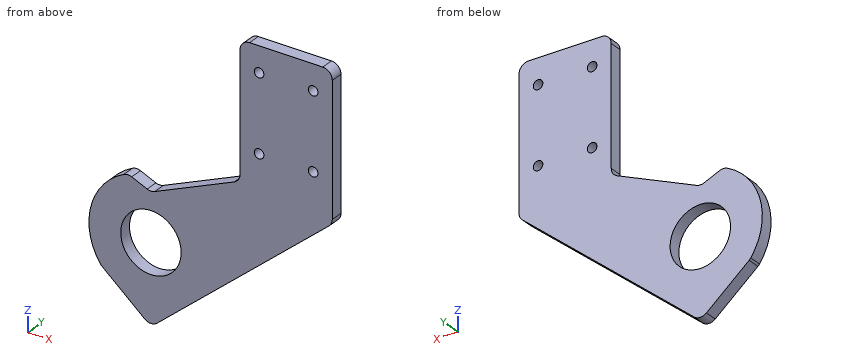
```python
from build123d import *

# Parameters (mm, degrees)
SKETCH_2_R          = 1.5
SKETCH_2_R_2        = 9.5
EXTRUDE_1_DEPTH     = 4
CUT_EXTRUDE_1_DEPTH = 124.429075185
SKETCH_6_R          = 1.5
EXTRUDE_2_DEPTH     = 4
FILLET_1_R          = 3


with BuildPart() as part:
    # 草图2 → 凸台-拉伸1 (new body)
    with BuildSketch(Plane(origin=(0, 0, 0), x_dir=(1, 0, 0), z_dir=(0, 1, 0))):
        Polygon((0, 0), (0, 60), (40, 93.908128514), (80, 60), (80, 0), (68, 0), (68, 42), (40, 54), (12, 42), (12, 0), align=None)
        with Locations(Location((6, 32, 0), (0, 0, 270))):
            Circle(SKETCH_2_R, mode=Mode.SUBTRACT)
        with Locations(Location((6, 8, 0), (0, 0, 270))):
            Circle(SKETCH_2_R, mode=Mode.SUBTRACT)
        with Locations(Location((40, 69, 0), (0, 0, 270))):
            Circle(SKETCH_2_R_2, mode=Mode.SUBTRACT)
        with Locations(Location((74, 8, 0), (0, 0, 90))):
            Circle(SKETCH_2_R, mode=Mode.SUBTRACT)
        with Locations(Location((74, 32, 0), (0, 0, 90))):
            Circle(SKETCH_2_R, mode=Mode.SUBTRACT)
    extrude(amount=EXTRUDE_1_DEPTH)

    # 草图4 → 切除-拉伸1 (cut, through all)
    with BuildSketch(Plane(origin=(0, 4, 0), x_dir=(1, 0, 0), z_dir=(0, 1, 0))):
        with BuildLine():
            Line((24.36723091, 80.656179931), (0, 60))
            Line((0, 60), (0, 0))
            Line((0, 0), (12, 0))
            Line((12, 0), (12, 42))
            Line((12, 42), (32.756034747, 50.895443463))
            ThreePointArc((32.756034747, 50.895443463), (21.23136653, 63.709593809), (24.36723091, 80.656179931))
        make_face()
    extrude(amount=-CUT_EXTRUDE_1_DEPTH, mode=Mode.SUBTRACT)

    # 草图6 → 凸台-拉伸2 (add)
    with BuildSketch(Plane(origin=(0, 4, 0), x_dir=(1, 0, 0), z_dir=(0, 1, 0))):
        Polygon((97, 45.589045381), (80, 60), (80, 0), (97, 0), align=None)
        with Locations(Location((91, 8, 0), (0, 0, 270))):
            Circle(SKETCH_6_R, mode=Mode.SUBTRACT)
        with Locations(Location((91, 32, 0), (0, 0, 270))):
            Circle(SKETCH_6_R, mode=Mode.SUBTRACT)
    extrude(amount=-EXTRUDE_2_DEPTH)

    # 圆角1
    fillet_1_edges = [part.edges().sort_by_distance(p)[0] for p in [
        (40, 2, -93.908128514),
        (68, 2, 0),
        (68, 2, -42),
        (40, 2, -54),
        (24.36723091, 2, -80.656179931),
        (32.756034747, 2, -50.895443463),
        (97, 2, -45.589045381),
        (97, 2, 0),
    ]]
    fillet(fillet_1_edges, radius=FILLET_1_R)


solid = part.part
```
Geometry check sheet. Reference: the model listing, model coordinates, mm. Give positions to 0.01 mm unless a question says otherwise; leave off trailing zeros. Write each loop counter-clockwise with the first axis right and the second up, starting at its lowest first coordinate (ties: lowest second). Pieces come first, ordered by that corner, then holes. Notation, with made-up numbers: (23, -15.5) - (52, -15.5) arc R21 ccw to (52, 4.5) - close; hole circle Ø6 at (39.5, 62). An arc over 180 degrees is marked (long way). Use a Markdown table: item, result.
Q1. Section check D-D, the plane y = 3.3. Enter the section's corners in (x, z).
Computed:
| item | result |
|---|---|
| outline | (24.14, -80.34) arc R3 ccw to (24.64, -80.89) - (38.06, -92.26) arc R3 ccw to (41.94, -92.26) - (95.94, -46.49) arc R3 ccw to (97, -44.2) - (97, -3) arc R3 ccw to (94, 0) - (71, 0) arc R3 ccw to (68, -3) - (68, -40.02) arc R3 cw to (66.18, -42.78) - (41.18, -53.49) arc R3 cw to (38.82, -53.49) - (33.96, -51.41) arc R3 ccw to (31.46, -51.47) arc R19.5 ccw to start; hole circle Ø19 at (40, -69); hole circle Ø3 at (74, -32); hole circle Ø3 at (74, -8); hole circle Ø3 at (91, -32); hole circle Ø3 at (91, -8) |
Q2. Section check B-B, the plane x = 40. Enter the section's corners in (y, z).
Computed:
| item | result |
|---|---|
| outline | (0, -92.98) - (4, -92.98) - (4, -78.5) - (0, -78.5) - close; (0, -59.5) - (4, -59.5) - (4, -53.74) - (0, -53.74) - close |
Q3. Section check C-C, the plane z = -62. Enter the section's corners in (x, y), then the cut area to 3 significant figures.
Computed:
| item | result |
|---|---|
| outline | (21.8, 0) - (33.58, 0) - (33.58, 4) - (21.8, 4) - close; (46.42, 0) - (77.64, 0) - (77.64, 4) - (46.42, 4) - close |
| area | 172 mm² |
Q4. Section check A-A, the plane z = -32. Enter the section's corners in (x, y).
Computed:
| item | result |
|---|---|
| outline | (68, 0) - (72.5, 0) - (72.5, 4) - (68, 4) - close; (75.5, 0) - (89.5, 0) - (89.5, 4) - (75.5, 4) - close; (92.5, 0) - (97, 0) - (97, 4) - (92.5, 4) - close |
Q5. Go/stop test with flat-tipped pins: P1, Ø15, axis at x = 40, z = -69, coming from the +Y side; P2, Ø1.2, axis at y = 2.5, z = -19, coming from the -X side; P3, Ø1.5, axis at x = 30.5, y = 3.5, coming from the +Z side. Record where each tip stops, or that it passes through.
Computed:
| item | result |
|---|---|
| P1 | passes through |
| P2 | stops at x = 68 |
| P3 | stops at z = -51.57 |
Q6. Thickness scan on L1, parallel to X at y = 1.85, z = -8; L2, parallel to Z at x = 74, y = 1.3; L3, parallel to X at y = 2.2, z = -7. Record the ranges inside material, lowest first. Write a range as [from, to].
Computed:
| item | result |
|---|---|
| L1 | x = [68, 72.5], [75.5, 89.5], [92.5, 97] |
| L2 | z = [-65.09, -33.5], [-30.5, -9.5], [-6.5, 0] |
| L3 | x = [68, 72.88], [75.12, 89.88], [92.12, 97] |
